The model under review builds one solid part; all positions refer to its coordinate system, in mm. Face numbers are marked on the shaded views. Round coordinates to 2 decimals unless told otherwise and drop trailing zeros. Order: outer loops, then holes, each group sorted by start corner. A loop starts at its lowest first (then second) coordinate and runs counter-clockwise, first axis right, second up.
```python
from build123d import *

# Parameters (mm, degrees)
CROQUIS1_W              = 95
CROQUIS1_H              = 59.2
SALIENTE_EXTRUIR1_DEPTH = 1
CROQUIS2_W              = 85.6
CROQUIS2_H              = 56.3
SALIENTE_EXTRUIR2_DEPTH = 3.4
CROQUIS3_W              = 74
CROQUIS3_H              = 49.3
CORTAR_EXTRUIR1_DEPTH   = 1
CROQUIS4_R              = 1.5
CORTAR_EXTRUIR2_DEPTH   = 11
CROQUIS5_R              = 0.5
CORTAR_EXTRUIR3_DEPTH   = 10


with BuildPart() as part:
    # Croquis1 → Saliente-Extruir1 (new body)
    with BuildSketch(Plane(origin=(0, 0, 0), x_dir=(1, 0, 0), z_dir=(0, 1, 0))):
        Rectangle(CROQUIS1_W, CROQUIS1_H)
    extrude(amount=SALIENTE_EXTRUIR1_DEPTH)

    # Croquis2 → Saliente-Extruir2 (add)
    with BuildSketch(Plane(origin=(0, 1, 0), x_dir=(1, 0, 0), z_dir=(0, 1, 0))):
        Rectangle(CROQUIS2_W, CROQUIS2_H)
    extrude(amount=SALIENTE_EXTRUIR2_DEPTH)

    # Croquis3 → Cortar-Extruir1 (cut)
    with BuildSketch(Plane(origin=(0, 4.4, 0), x_dir=(1, 0, 0), z_dir=(0, 1, 0))):
        with Locations((-2.3, 0)):
            Rectangle(CROQUIS3_W, CROQUIS3_H)
    extrude(amount=-CORTAR_EXTRUIR1_DEPTH, mode=Mode.SUBTRACT)

    # Croquis4 → Cortar-Extruir2 (cut)
    with BuildSketch(Plane(origin=(0, 1, 0), x_dir=(1, 0, 0), z_dir=(0, 1, 0))):
        with Locations(Location((45, -23.8, 0), (0, 0, 270))):
            Circle(CROQUIS4_R)
        with Locations(Location((45, 23.8, 0), (0, 0, 90))):
            Circle(CROQUIS4_R)
        with Locations(Location((-45, -23.8, 0), (0, 0, 90))):
            Circle(CROQUIS4_R)
        with Locations(Location((-45, 23.8, 0), (0, 0, 270))):
            Circle(CROQUIS4_R)
    extrude(amount=-CORTAR_EXTRUIR2_DEPTH, mode=Mode.SUBTRACT)

    # Croquis5 → Cortar-Extruir3 (cut)
    with BuildSketch(Plane(origin=(0, 1, 0), x_dir=(1, 0, 0), z_dir=(0, 1, 0))):
        with Locations(Location((-45.35, -9.63, 0), (0, 0, 270))):
            Circle(CROQUIS5_R)
        with Locations(Location((-45.35, -7.09, 0), (0, 0, 270))):
            Circle(CROQUIS5_R)
        with Locations(Location((-45.35, -4.55, 0), (0, 0, 270))):
            Circle(CROQUIS5_R)
        with Locations(Location((-45.35, -2.01, 0), (0, 0, 270))):
            Circle(CROQUIS5_R)
        with Locations(Location((-45.35, 0.53, 0), (0, 0, 270))):
            Circle(CROQUIS5_R)
        with Locations(Location((-45.35, 3.07, 0), (0, 0, 270))):
            Circle(CROQUIS5_R)
        with Locations(Location((-45.35, 5.61, 0), (0, 0, 270))):
            Circle(CROQUIS5_R)
        with Locations(Location((-45.35, 8.15, 0), (0, 0, 270))):
            Circle(CROQUIS5_R)
        with Locations(Location((-45.35, 10.69, 0), (0, 0, 270))):
            Circle(CROQUIS5_R)
    extrude(amount=-CORTAR_EXTRUIR3_DEPTH, mode=Mode.SUBTRACT)


solid = part.part
```
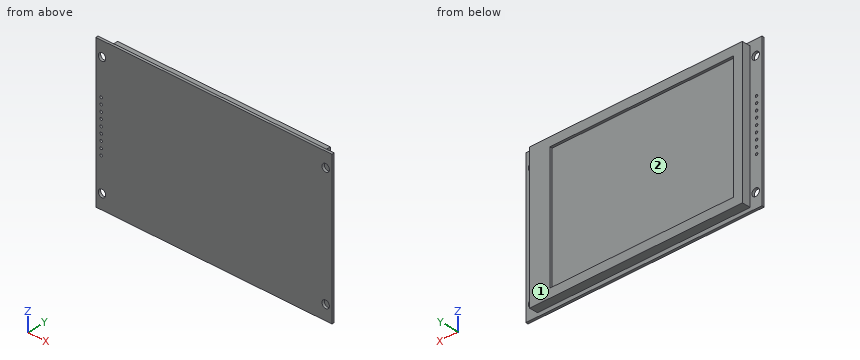
(1) Consider section C-C (x = 3.5). Write out the cut boundary in (y, z), and give its area (3 significant figures).
Data:
outline: (0, -29.6) - (1, -29.6) - (1, -28.15) - (4.4, -28.15) - (4.4, -24.65) - (3.4, -24.65) - (3.4, 24.65) - (4.4, 24.65) - (4.4, 28.15) - (1, 28.15) - (1, 29.6) - (0, 29.6) - close
area: 201 mm2
(2) Draft analysis for pull direction Z (two halves, no side actions). For the marked faces 1 and 2, state which applies: pulls with the +Z half, pulls with the -Z half, needs draft (parallel to the pull), parting line crosses it, or undercut.
Data:
face 1: needs draft
face 2: undercut
(3) Consider section D-D (y = 2.05). Write out the cut boundary in (x, z).
Data:
outline: (-42.8, -28.15) - (42.8, -28.15) - (42.8, 28.15) - (-42.8, 28.15) - close
(4) Insertion check: pin 1 (12 mm diameter, centred on x = 5.5, z = 17.5, fed in from -Y); pin 2 (1 mm diameter, centred on y = 3.5, z = -17, fed in from -X); pin 3 (0.8 mm diameter, centred on y = 4, z = -5.5, fed in from +X); pin 4 (1.7 mm diameter, centred on x = -17, y = 2.5, fed in from -Z). Each pin has a flat end and moves straight along its axis. Give the tip position at first contact, or say it passes through.
Data:
pin 1: stops at y = 0
pin 2: stops at x = -42.8
pin 3: stops at x = 42.8
pin 4: stops at z = -28.15
(5) Consider section B-B (z = -17). Write out the cut boundary in (x, y).
Data:
outline: (-47.5, 0) - (47.5, 0) - (47.5, 1) - (42.8, 1) - (42.8, 4.4) - (34.7, 4.4) - (34.7, 3.4) - (-39.3, 3.4) - (-39.3, 4.4) - (-42.8, 4.4) - (-42.8, 1) - (-47.5, 1) - close
(6) To check wall thickness, follow probe 1 along X at (y, z) = (3.6, -5); probe 2 along Z at (x, y) = (23, 4.15); probe 3 along X at (y, z) = (0.4, 4.55). State the ranges of each line that lie inside material, in increasing order.
Data:
probe 1: x = -42.8 to -39.3, 34.7 to 42.8
probe 2: z = -28.15 to -24.65, 24.65 to 28.15
probe 3: x = -47.5 to -45.85, -44.85 to 47.5
(7) Consider section A-A (x = 45). Write out the cut boundary in (y, z), and give its area (3 significant figures).
Data:
outline: (0, -29.6) - (1, -29.6) - (1, -25.3) - (0, -25.3) - close; (0, -22.3) - (1, -22.3) - (1, 22.3) - (0, 22.3) - close; (0, 25.3) - (1, 25.3) - (1, 29.6) - (0, 29.6) - close
area: 53.2 mm2
